The drawing under review shows one solid part. Ordinate dimensions are in mm from its lowest x, y, z. Round coordinates to 2 decimals unless told otherwise and drop trailing zeros. Write each loop counter-clockwise with the first axis right and the second up, starting at its lowest first coordinate (ties: lowest second). Pieces come first, ordered by that corner, then holes. Notation, with made-up numbers: (69, 73.25) -> (126, 73.25) arc R23 cw to (126, 110.25) -> close; hole circle Ø3 at (-35.75, 81). An arc over 180 degrees is marked (long way). Answer in a Markdown table with one row per item. Add a question column.
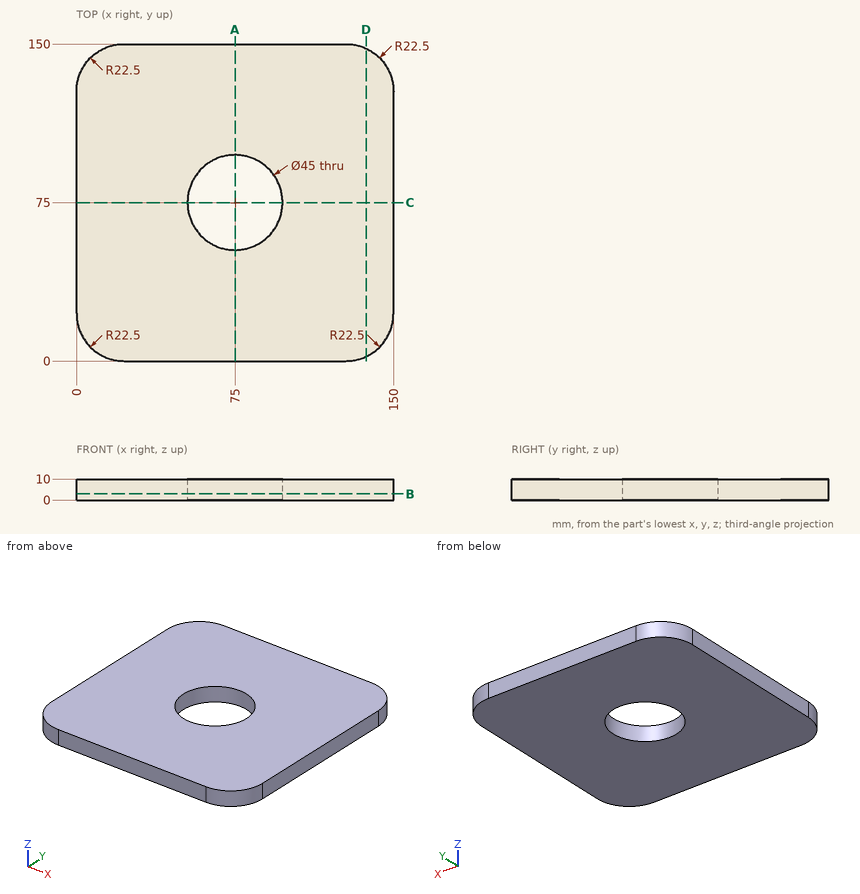
1. For L1, parallel to Y at x = 75, z = 3.75; L2, parallel to X at y = 87.5, z = 7.75; L3, parallel to X at y = 78, z = 4.25, list the stretches that pass through material, from the lowest coordinate up.
2. Add section B-B on z = 3. Write out the cut boundary in (x, y), plus the area to 3 significant figures.
3. Add section A-A on x = 75. Write out the cut boundary in (y, z).
4. Add section D-D on x = 137. Write out the cut boundary in (y, z), plus the area to 3 significant figures.
Filled in:
| question | item | result |
|---|---|---|
| 1 | L1 | 0 to 52.5, 97.5 to 150 |
| 1 | L2 | 0 to 56.29, 93.71 to 150 |
| 1 | L3 | 0 to 52.7, 97.3 to 150 |
| 2 | outline | (0, 22.5) arc R22.5 ccw to (22.5, 0) -> (127.5, 0) arc R22.5 ccw to (150, 22.5) -> (150, 127.5) arc R22.5 ccw to (127.5, 150) -> (22.5, 150) arc R22.5 ccw to (0, 127.5) -> close; hole circle Ø45 at (75, 75) |
| 2 | area | 20,500 mm² |
| 3 | outline | (0, 0) -> (52.5, 0) -> (52.5, 10) -> (0, 10) -> close; (97.5, 0) -> (150, 0) -> (150, 10) -> (97.5, 10) -> close |
| 4 | outline | (2.1, 0) -> (147.9, 0) -> (147.9, 10) -> (2.1, 10) -> close |
| 4 | area | 1,460 mm² |
